from build123d import *

# Parameters (mm, degrees)
SKETCH23_W           = 55.7
SKETCH23_H           = 37.7
SKETCH23_W_2         = 47.7
SKETCH23_H_2         = 29.7
BOSS_EXTRUDE11_DEPTH = 34.1
BOSS_EXTRUDE3_DEPTH  = 4.5
SKETCH19_W           = 4.5
SKETCH19_H           = 20
SKETCH19_W_2         = 20
SKETCH19_H_2         = 4.5
SKETCH19_W_3         = 8
SKETCH19_H_3         = 38.319745762
SKETCH19_W_4         = 16.618093031
SKETCH19_H_4         = 8
BOSS_EXTRUDE10_DEPTH = 16
FILLET6_R            = 16
FILLET7_R            = 2
SKETCH11_R           = 1.2
CUT_EXTRUDE1_DEPTH   = 111.325510764
SKETCH21_R           = 2.35
CUT_EXTRUDE2_DEPTH   = 2.4
SKETCH22_R           = 2.35
CUT_EXTRUDE3_DEPTH   = 2.4


with BuildPart() as part:
    # Sketch23 → Boss-Extrude11 (new body)
    with BuildSketch(Plane(origin=(0, 0, 0), x_dir=(1, 0, 0), z_dir=(0, 1, 0))):
        with Locations((27.85, -18.85)):
            Rectangle(SKETCH23_W, SKETCH23_H)
        with Locations((27.85, -18.85)):
            Rectangle(SKETCH23_W_2, SKETCH23_H_2, mode=Mode.SUBTRACT)
    extrude(amount=-BOSS_EXTRUDE11_DEPTH)

    # Sketch12 → Boss-Extrude3 (add)
    with BuildSketch(Plane(origin=(0, 0, 0), x_dir=(1, 0, 0), z_dir=(0, 1, 0))):
        Polygon((0, -76.019745762), (-12.2428, -76.019745762), (-16.7428, -76.019745762), (-16.7428, -56.019745762), (-12.2428, -56.019745762), (0, -56.019745762), (8, -56.019745762), (8, -76.019745762), align=None)
        Polygon((52.318093031, -8), (52.318093031, 0), (52.318093031, 12.2428), (52.318093031, 16.7428), (72.318093031, 16.7428), (72.318093031, 12.2428), (72.318093031, 0), (72.318093031, -8), align=None)
    extrude(amount=BOSS_EXTRUDE3_DEPTH)


with BuildPart() as boss_extrude3_piece_1:
    # of the separate pieces the step leaves, piece 1, a body of its own (boss_extrude3_pieces)
    add(part.part.solids().sort_by_distance((0, 0, 0))[0])



with BuildPart() as boss_extrude3_piece_2:
    # of the separate pieces the step leaves, piece 2, a body of its own (boss_extrude3_pieces)
    add(part.part.solids().sort_by_distance((8, 0, 76.019745762))[0])


with BuildPart() as boss_extrude3_piece_1_1:
    add(boss_extrude3_piece_1.part)

    add(boss_extrude3_piece_2.part)  # Boss-Extrude10 merges Boss-Extrude3 piece 2
    # Sketch19 → Boss-Extrude10 (add)
    with BuildSketch(Plane(origin=(0, 0, 0), x_dir=(1, 0, 0), z_dir=(0, 1, 0))):
        with Locations((-14.4928, -66.019745762)):
            Rectangle(SKETCH19_W, SKETCH19_H)
        with Locations((62.318093031, 14.4928)):
            Rectangle(SKETCH19_W_2, SKETCH19_H_2)
        with Locations((4, -56.859872881)):
            Rectangle(SKETCH19_W_3, SKETCH19_H_3)
        with Locations((64.009046516, -4)):
            Rectangle(SKETCH19_W_4, SKETCH19_H_4)
    extrude(amount=-BOSS_EXTRUDE10_DEPTH)

    # Fillet6
    fillet6_edges = [boss_extrude3_piece_1_1.edges().sort_by_distance(p)[0] for p in [
        (72.318093031, -16, 4),
        (4, -16, 76.019745762),
    ]]
    fillet(fillet6_edges, radius=FILLET6_R)

    # Fillet7
    fillet7_edges = [boss_extrude3_piece_1_1.edges().sort_by_distance(p)[0] for p in [
        (67.63180153, -11.313708499, 8),
        (8, 2.25, 76.019745762),
        (8, -16, 48.859872881),
        (8, -11.313708499, 71.333454261),
        (55.7, -34.1, 18.85),
        (72.318093031, 2.25, 8),
        (72.318093031, -5.75, -16.7428),
        (52.318093031, -5.75, -16.7428),
        (62.318093031, 4.5, 8),
        (72.318093031, 4.5, -4.3714),
        (62.318093031, 4.5, -16.7428),
        (52.318093031, 4.5, -4.3714),
        (-16.7428, -5.75, 56.019745762),
        (-16.7428, -5.75, 76.019745762),
        (8, 4.5, 66.019745762),
        (-4.3714, 4.5, 56.019745762),
        (-16.7428, 4.5, 66.019745762),
        (-4.3714, 4.5, 76.019745762),
        (56.009046515, -16, 8),
        (-16.7428, -16, 66.019745762),
        (55.7, -17.05, 37.7),
        (27.85, -34.1, 37.7),
        (62.318093031, -16, -16.7428),
    ]]
    fillet(fillet7_edges, radius=FILLET7_R)

    # Sketch11 → Cut-Extrude1 (cut, through all)
    with BuildSketch(Plane(origin=(0, 0, 0), x_dir=(-1, 0, 0), z_dir=(0, 0, -1))):
        with Locations(Location((-19.011079079, -11, 0), (0, 0, 180))):
            Circle(SKETCH11_R)
        with Locations(Location((-19.011079079, -23, 0), (0, 0, 180))):
            Circle(SKETCH11_R)
        with Locations(Location((-43.01107908, -11, 0), (0, 0, 180))):
            Circle(SKETCH11_R)
        with Locations(Location((-43.011079079, -23, 0), (0, 0, 180))):
            Circle(SKETCH11_R)
    extrude(amount=-CUT_EXTRUDE1_DEPTH, mode=Mode.SUBTRACT)

    # Sketch21 → Cut-Extrude2 (cut)
    with BuildSketch(Plane.XY.offset(37.7)):
        with Locations((19.011079079, -11)):
            Circle(SKETCH21_R)
        with Locations((43.01107908, -11)):
            Circle(SKETCH21_R)
        with Locations((19.011079079, -23)):
            Circle(SKETCH21_R)
        with Locations((43.011079079, -23)):
            Circle(SKETCH21_R)
    extrude(amount=-CUT_EXTRUDE2_DEPTH, mode=Mode.SUBTRACT)

    # Sketch22 → Cut-Extrude3 (cut)
    with BuildSketch(Plane(origin=(0, 0, 0), x_dir=(-1, 0, 0), z_dir=(0, 0, -1))):
        with Locations(Location((-43.01107908, -11, 0), (0, 0, 180))):
            Circle(SKETCH22_R)
        with Locations(Location((-43.011079079, -23, 0), (0, 0, 180))):
            Circle(SKETCH22_R)
        with Locations(Location((-19.011079079, -11, 0), (0, 0, 180))):
            Circle(SKETCH22_R)
        with Locations(Location((-19.011079079, -23, 0), (0, 0, 180))):
            Circle(SKETCH22_R)
    extrude(amount=-CUT_EXTRUDE3_DEPTH, mode=Mode.SUBTRACT)


solid = boss_extrude3_piece_1_1.part
Geometry check sheet. Reference: the model listing, model coordinates, mm. A direction names the side the tool comes from. Coordinates: 2 decimals unless noted, no trailing zeros. Loops run counter-clockwise (first coordinate to the right, second up) from the corner with the lowest first, then second, coordinate; pieces in that order, holes last. Notation, with made-up numbers: (88, 39) - (95, 39) arc R8 cw to (95, 45) - close; hole circle Ø4 at (-39.75, -21.75). An arc over 180 degrees is marked (long way). Use one line per item in the form item = value. Start each with the question number.
Item 1: Gauge pin test, flat ends, axial feed: pin 1 (13 mm diameter, centred on y = -8, z = 69.5, fed in from +X); pin 2 (2.5 mm diameter, centred on x = 19.5, y = -11, fed in from +Z); pin 3 (9 mm diameter, centred on y = -3.5, z = -4, fed in from -X); pin 4 (1.9 mm diameter, centred on x = 19.01, y = -11, fed in from +Z). Record the tip position at first contact, or that the pin passes through.
Item 2: Mould release check, pull along Y, two halves, no side actions. Record for faces 1 (the face through (55.7, -16, 18)), 2 (the face through (42, -12, 2.4)), 3 (the face through (62, 0, -6)): +Y half, -Y half, draft (parallel to the pull), parting line (faces both ways), or undercut.
Item 3: Section check D-D, the plane y = -7.5. Give the number of separate pieces and of enclosed holes in the cut face, and give its area (3 significant figures).
Item 4: Section check B-B, the plane y = -29. Enter the section's corners in (x, z), and give its area (3 significant figures).
Item 5: Section check C-C, the plane x = -3.5. Enter the section's corners in (y, z), and give its area (3 significant figures).
Item 6: Tool access check on faces 4 (the face through (0, -13, 30)), 5 (the face through (28, -17, 4)), 6 (the face through (62, -8, -12.243)), 7 (the face through (18, -22, 35.3)), 8 (the face through (42, -24, 2.4)). Record the directions out of +Z, -Z, +X, -X, +Y, -Y that give a thin tool (end or side, any length) a straight path to the whole face; none if there is none.
Item 7: Section check A-A, the plane z = 11. Enter the section's corners in (x, y), and give its area (3 significant figures).
Item 8: Thickness scan on probe 1 along X at (y, z) = (-11, 34.45); probe 2 along Z at (x, y) = (9.5, -21); probe 3 along X at (y, z) = (-11, 2.8). Record the ranges inside material, lowest first.
Computed:
q1.pin_1 = 8
q1.pin_2 = 35.3
q1.pin_3 = 0
q1.pin_4 = through
q2.face_1 = draft
q2.face_2 = undercut
q2.face_3 = -Y half
q3.separate_pieces = 3
q3.enclosed_holes = 1
q3.area = 1,270 mm2
q4.outline = (0, 0) - (55.7, 0) - (55.7, 35.7) arc R2 ccw to (53.7, 37.7) - (0, 37.7) - close; hole (4, 4) - (51.7, 4) - (51.7, 33.7) - (4, 33.7) - close
q4.area = 682 mm2
q5.outline = (0, 56.02) - (2.5, 56.02) arc R2 ccw to (4.5, 58.02) - (4.5, 74.02) arc R2 ccw to (2.5, 76.02) - (0, 76.02) - close
q5.area = 88.3 mm2
q6.face_4 = +Z, -Z, -Y
q6.face_5 = +Y, -Y
q6.face_6 = +X, -X, -Y
q6.face_7 = +Z
q6.face_8 = -Z
q7.outline = (0, -34.1) - (4, -34.1) - (4, 0) - (0, 0) - close; (51.7, -34.1) - (53.7, -34.1) arc R2 ccw to (55.7, -32.1) - (55.7, 0) - (51.7, 0) - close
q7.area = 272 mm2
q8.probe_1 = 0 to 17.81, 20.21 to 41.81, 44.21 to 55.7
q8.probe_2 = 0 to 4, 33.7 to 37.7
q8.probe_3 = 0 to 17.81, 20.21 to 41.81, 44.21 to 67.94
